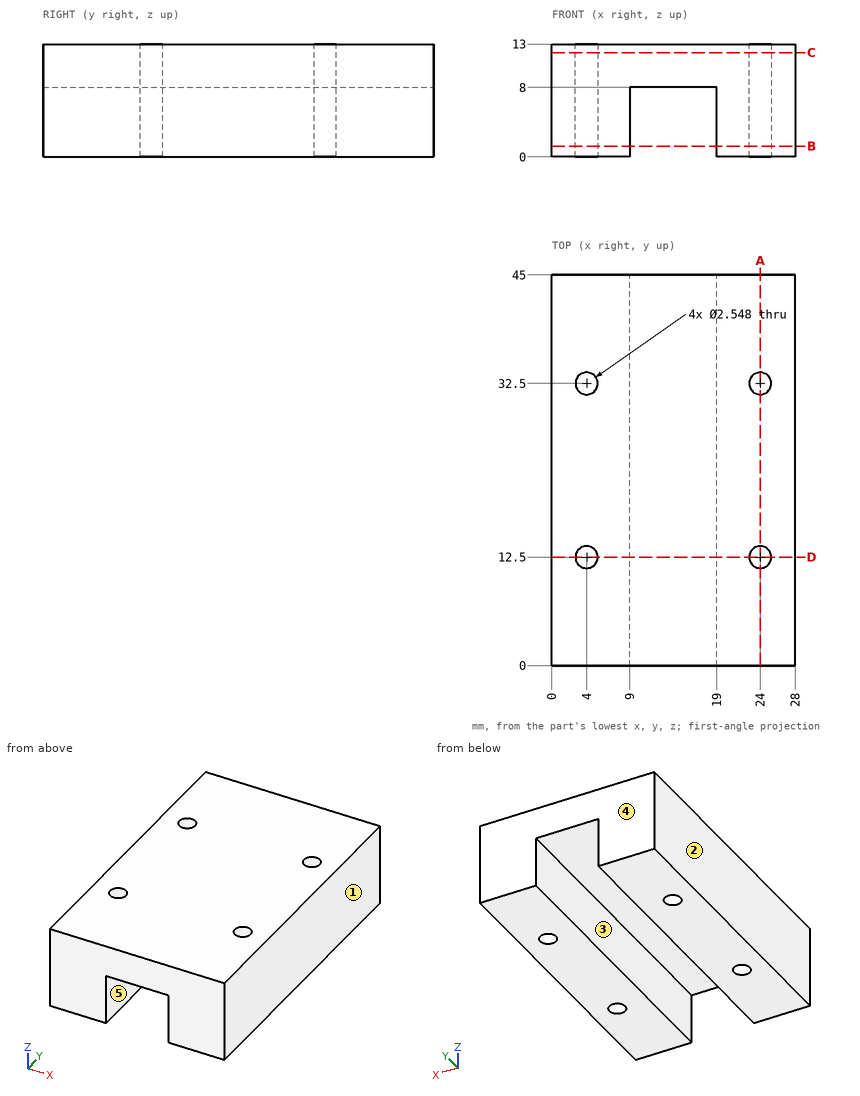
Source: three-view drawing plus pictorial views. Frame: mm from the lowest corner of the part. A direction names the side the tool comes from. Round coordinates to 2 decimals unless told otherwise and drop trailing zeros. Write each loop counter-clockwise with the first axis right and the second up, starting at its lowest first coordinate (ties: lowest second). Pieces come first, ordered by that corner, then holes. Notation, with made-up numbers: M 61.25,37.5 L 67.25,37.5 A20 ccw 67.25,68.5 Z; hole C -20.5,49.5 d7. An arc over 180 degrees is marked long. One line per item, written item: value. Start each with the question number.
Item 1: Set-up query: the marked faces 4 and 5. Return all of +Z, -Z, +X, -X, +Y, -Y with unobstructed straight access to the full face (end or side cutting, diameter ignored); none if empty.
Item 2: Section query B-B (z = 1.25). Return the cut outline in (x, y).
Item 3: Section query A-A (x = 24). Return the cut outline in (y, z).
Item 4: Ray query, L1, parallel to Y at x = 4, z = 8; L2, parallel to X at y = 16.5, z = 2.75; L3, parallel to X at y = 32, z = 6.5. Return the intervals inside material, ascending. Write a range as from..to.
Item 5: Mould query, pull axis X, two halves, no side actions, for the marked faces 1, 2 and 3. Classes: pulls with the +X half, pulls with the -X half, needs draft (parallel to the pull), parting line crosses it, or undercut.
Item 6: Section query C-C (z = 12). Return the cut outline in (x, y), plus the area to 3 significant figures.
Item 7: Pin query (flat end, axial travel): pin 1 (1.5 mm diameter, centred on x = 24, y = 32.5, fed in from -Z). Return the tip coordinate at first contact, or that it passes through.
Item 8: Section query D-D (y = 12.5). Return the cut outline in (x, z), plus the area to 3 significant figures.
Result set:
1. face 4: +Z, -Z, +X, -X, +Y
1. face 5: -Z, +Y, -Y
2. outline: M 0,0 L 9,0 L 9,45 L 0,45 Z; M 19,0 L 28,0 L 28,45 L 19,45 Z; hole C 4,12.5 d2.55; hole C 4,32.5 d2.55; hole C 24,12.5 d2.55; hole C 24,32.5 d2.55
3. outline: M 0,0 L 11.23,0 L 11.23,13 L 0,13 Z; M 13.77,0 L 31.23,0 L 31.23,13 L 13.77,13 Z; M 33.77,0 L 45,0 L 45,13 L 33.77,13 Z
4. L1: y = 0..11.23, 13.77..31.23, 33.77..45
4. L2: x = 0..9, 19..28
4. L3: x = 0..2.83, 5.17..9, 19..22.83, 25.17..28
5. face 1: pulls with the +X half
5. face 2: pulls with the -X half
5. face 3: undercut
6. outline: M 0,0 L 28,0 L 28,45 L 0,45 Z; hole C 4,12.5 d2.55; hole C 4,32.5 d2.55; hole C 24,12.5 d2.55; hole C 24,32.5 d2.55
6. area: 1,240 mm²
7. pin 1: passes through
8. outline: M 0,0 L 2.73,0 L 2.73,13 L 0,13 Z; M 5.27,0 L 9,0 L 9,8 L 19,8 L 19,0 L 22.73,0 L 22.73,13 L 5.27,13 Z; M 25.27,0 L 28,0 L 28,13 L 25.27,13 Z
8. area: 218 mm²
